from build123d import *

# Parameters (mm, degrees)
F0_R     = 34.5
F1_DEPTH = 13
F1_TAPER = -8.75
F2_R     = 42.5
F3_DEPTH = 2
F3_TAPER = -8.7
F4_R     = 2


with BuildPart() as f1:
    # F0 (on Top) → F1 (new body)
    with BuildSketch(Plane.XY):
        Circle(F0_R)
    extrude(amount=F1_DEPTH, taper=F1_TAPER)

    # F2 (on face) → F3 (join)
    with BuildSketch(Plane.XY.offset(13)):
        Circle(F2_R)
    extrude(amount=F3_DEPTH, taper=F3_TAPER)

    # F4
    f4_edges = [f1.edges().sort_by_distance(p)[0] for p in [
        (-34.5, 0, 0),
        (-36.500891, 0, 13),
        (-42.5, 0, 13),
    ]]
    fillet(f4_edges, radius=F4_R)


solid = f1.part
The model under review builds one solid part; all positions refer to its coordinate system, in mm. A direction names the side the tool comes from. Round coordinates to 2 decimals unless told otherwise and drop trailing zeros. Order: outer loops, then holes, each group sorted by start corner. A loop starts at its lowest first (then second) coordinate and runs counter-clockwise, first axis right, second up. Notation, with made-up numbers: (-28, 37.5) -> (7, 37.5) arc R22 ccw to (7, 72.5) -> close; hole circle Ø3 at (-3, 10.25). An arc over 180 degrees is marked (long way). Write item = value, one per line. Start each with the question number.
Item 1: For line 1 along Z through (x, y) = (-27.5, -28.5); line 2 along X through (y, z) = (3.5, 5); line 3 along X through (y, z) = (-5.5, 12), list the stretches that pass through material, from the lowest coordinate up.
Item 2: For faces 1 (the face through (-12.3, 36.4, 13)), 2 (the face through (0, 0, 0)), list the 3-axis set-ups (+Z, -Z, +X, -X, +Y, -Y) from which the entire face can be reached by the end or side of a thin tool; tool diameter is ignored.
Item 3: Consider section C-C on z = 9.25. Write out the cut boundary in (x, y).
Item 4: Clearance check with flat-ended pins moving along their axes: pin 1 Ø6 at (x, z) = (26, 7.5) entering from +Y; pin 2 Ø5 at (y, z) = (23.5, 1.5) entering from -X; pin 3 Ø4 at (y, z) = (-25.5, 2.5) entering from +X. State where each tip first meets the part, or that it passes through.
Item 5: Consider section A-A on x = 0. Write out the cut boundary in (y, z).
Item 6: Consider section B-B on z = 4.5. Write out the cut boundary in (x, y).
Conclusion:
q1.line_1 = 13 to 15
q1.line_2 = -35.1 to 35.1
q1.line_3 = -36.07 to 36.07
q2.face_1 = -Z
q2.face_2 = -Z, +X, -X, +Y, -Y
q3.outline = circle Ø71.85 at (0, 0)
q4.pin_1 = 27.32
q4.pin_2 = -27.72
q4.pin_3 = 25.83
q5.outline = (-42.81, 15) -> (-42.76, 14.7) arc R2 ccw to (-40.78, 13) -> (-38.22, 13) arc R2 cw to (-36.24, 11.3) -> (-34.76, 1.7) arc R2 ccw to (-32.78, 0) -> (32.78, 0) arc R2 ccw to (34.76, 1.7) -> (36.24, 11.3) arc R2 cw to (38.22, 13) -> (40.78, 13) arc R2 ccw to (42.76, 14.7) -> (42.81, 15) -> close
q6.outline = circle Ø70.39 at (0, 0)
